Read the model definition and answer for the solid it produces. Units are mm, in the model's axes. A direction names the side the tool comes from. Coordinates: 2 decimals unless noted, no trailing zeros. Order: outer loops, then holes, each group sorted by start corner. A loop starts at its lowest first (then second) coordinate and runs counter-clockwise, first axis right, second up. Notation, with made-up numbers: (50.5, 82.25) - (83.5, 82.25) arc R37 cw to (83.5, 119.25) - close; hole circle Ø1 at (-26.5, 67). An arc over 180 degrees is marked (long way). Write item = value, one per line.
from build123d import *

# Parameters (mm, degrees)
AUFSATZ_LINEAR_AUSTRAGEN1_DEPTH = 3
SKIZZE2_R                       = 2
AUFSATZ_LINEAR_AUSTRAGEN2_DEPTH = 76


with BuildPart() as part:
    # Skizze1 → Aufsatz-Linear austragen1 (new body)
    with BuildSketch(Plane.XY):
        Polygon((-1.777039873, 0.285182154), (0.34428047, 2.406502498), (3.34428047, 2.406502498), (5.465600814, 0.285182154), (5.465600814, -2.714817846), (3.34428047, -4.83613819), (0.34428047, -4.83613819), (-1.777039873, -2.714817846), align=None)
    extrude(amount=AUFSATZ_LINEAR_AUSTRAGEN1_DEPTH)

    # Skizze2 → Aufsatz-Linear austragen2 (add)
    with BuildSketch(Plane.XY.offset(3)):
        with Locations((1.84428047, -1.214817846)):
            Circle(SKIZZE2_R)
    extrude(amount=AUFSATZ_LINEAR_AUSTRAGEN2_DEPTH)


solid = part.part
1) For faces 1 (the face through (4, 0, 3)), 2 (the face through (4.39, 1.36, 1.48)), determine the directions among +Z, -Z, +X, -X, +Y, -Y from which every point of the face is accessible in a straight line to the end or side of a thin tool.
Returned:
face_1 = +Z
face_2 = +Z, -Z, +X, +Y
2) The part is cut by section A-A (x = 2.25). Determine the outline of the cut face in (y, z), and give its area (3 significant figures).
Returned:
outline = (-4.84, 0) - (2.41, 0) - (2.41, 3) - (0.74, 3) - (0.74, 79) - (-3.17, 79) - (-3.17, 3) - (-4.84, 3) - close
area = 319 mm^2
3) Straight lines are drawn through the part: line 1 along Z through (x, y) = (4.75, -1.5); line 2 along Y through (x, z) = (1.75, 30.5); line 3 along X through (y, z) = (-3, 58). For each, find the intervals that lie inside material, in ascending order. Write a range as from..to.
Returned:
line_1 = 0..3
line_2 = -3.21..0.78
line_3 = 0.94..2.75
4) The part is cut by section D-D (x = -1). Determine the outline of the cut face in (y, z), and give its area (3 significant figures).
Returned:
outline = (-3.49, 0) - (1.06, 0) - (1.06, 3) - (-3.49, 3) - close
area = 13.7 mm^2
5) Flat-ended cylindrical pins translate along their axes: pin 1 Ø1 at (y, z) = (-2, 22) entering from +X; pin 2 Ø1.5 at (x, z) = (2, 70.5) entering from -Y. Find the tip coordinate at first contact, or state that the pin passes through.
Returned:
pin_1 = 3.82
pin_2 = -3.21
6) The part is cut by section B-B (y = -4). Determine the outline of the cut face in (x, z).
Returned:
outline = (-0.49, 0) - (4.18, 0) - (4.18, 3) - (-0.49, 3) - close
7) The part is cut by section C-C (z = 16.5). Determine the outline of the cut face in (x, y), and give its area (3 significant figures).
Returned:
outline = circle Ø4 at (1.84, -1.21)
area = 12.6 mm^2
